Model file for the job. Use its own axes, mm. A direction names the side the tool comes from. Give positions to 0.01 mm unless a question says otherwise; leave off trailing zeros. Loops run counter-clockwise (first coordinate to the right, second up) from the corner with the lowest first, then second, coordinate; pieces in that order, holes last. Notation, with made-up numbers: M 89,32 L 105,32 A23 ccw 105,54 Z; hole C 0.5,64 d5. An arc over 180 degrees is marked long. Answer in a Markdown table with one row per item.
```python
from build123d import *

# Parameters (mm, degrees)
F0_R     = 2.55
F1_DEPTH = 5


with BuildPart() as f1:
    # F0 (on Top) → F1 (new body)
    with BuildSketch(Plane.XY):
        Polygon((-61.291651, 58.480762), (-81.291651, 23.839746), (-20, -11.547005), (-20, -82.320508), (20, -82.320508), (20, -11.547005), (81.291651, 23.839746), (61.291651, 58.480762), (0, 23.094011), align=None)
        with Locations((-10, -72.320508)):
            Circle(F0_R, mode=Mode.SUBTRACT)
        with Locations((-10, -32.320508)):
            Circle(F0_R, mode=Mode.SUBTRACT)
        with Locations((10, -72.320508)):
            Circle(F0_R, mode=Mode.SUBTRACT)
        with Locations((10, -32.320508)):
            Circle(F0_R, mode=Mode.SUBTRACT)
        with Locations((-67.631397, 27.5)):
            Circle(F0_R, mode=Mode.SUBTRACT)
        with Locations((-32.990381, 7.5)):
            Circle(F0_R, mode=Mode.SUBTRACT)
        with Locations((-22.990381, 24.820508)):
            Circle(F0_R, mode=Mode.SUBTRACT)
        with Locations((-57.631397, 44.820508)):
            Circle(F0_R, mode=Mode.SUBTRACT)
        with Locations((32.990381, 7.5)):
            Circle(F0_R, mode=Mode.SUBTRACT)
        with Locations((22.990381, 24.820508)):
            Circle(F0_R, mode=Mode.SUBTRACT)
        with Locations((67.631397, 27.5)):
            Circle(F0_R, mode=Mode.SUBTRACT)
        with Locations((57.631397, 44.820508)):
            Circle(F0_R, mode=Mode.SUBTRACT)
    extrude(amount=F1_DEPTH)


solid = f1.part
```
(1) Saw through at B-B, the plane x = 10. Give the cut face in (y, z), and give its area (3 significant figures).
Established:
| item | result |
|---|---|
| outline | M -82.32,0 L -74.87,0 L -74.87,5 L -82.32,5 Z; M -69.77,0 L -34.87,0 L -34.87,5 L -69.77,5 Z; M -29.77,0 L 28.87,0 L 28.87,5 L -29.77,5 Z |
| area | 505 mm2 |
(2) Saw through at D-D, the plane y = -54.5. Give the cut face in (x, z).
Established:
| item | result |
|---|---|
| outline | M -20,0 L 20,0 L 20,5 L -20,5 Z |
(3) Flat gauge pins, fed straight in: P1, Ø3, axis at y = 14, z = 3, coming from the +X side; P2, Ø1, axis at y = -8.5, z = 2, coming from the -X side; P3, Ø1, axis at x = -63.5, z = 3, coming from the +Y side. Where does each tip first touch, or does it go through?
Established:
| item | result |
|---|---|
| P1 | stops at x = 66.85 |
| P2 | stops at x = -26.14 |
| P3 | stops at y = 55.52 |
(4) Mould opens along Y. For faces 1 (the flat face through (20, -47, 2)), 2 (the cylindrical face through (-24.87, 26.544, 2.465)), 3 (the cylindrical face through (11.37, -70.17, 2.46)), 4 (the flat face through (50.22, 5.9, 2.46)) say: pulls with the +Y half, pulls with the -Y half, needs draft (parallel to the pull), parting line crosses it, or undercut.
Established:
| item | result |
|---|---|
| face 1 | needs draft |
| face 2 | undercut |
| face 3 | undercut |
| face 4 | pulls with the -Y half |
(5) Which spindle directions (+Z, -Z, +X, -X, +Y, -Y) get a long thin tool onto all of the face, cutting with end or side? Do faces 5 (the flat face through (-20, -46, 2)), 6 (the flat face through (71.43, 40.92, 2.46)), 7 (the flat face through (-30.22, 40.54, 2.46)). Say none if no direction does.
Established:
| item | result |
|---|---|
| face 5 | +Z, -Z, -X, -Y |
| face 6 | +Z, -Z, +X, +Y |
| face 7 | +Z, -Z, +Y |
(6) Saw through at C-C, the plane z = 2.3. Count the separate pieces of the cut face and the enclosed holes in it, and give its area (3 significant figures).
Established:
| item | result |
|---|---|
| separate pieces | 1 |
| enclosed holes | 12 |
| area | 8,940 mm2 |
(7) Wall check: L1, parallel to X at y = 23, z = 1.55; L2, parallel to Y at x = -12, z = 4.55; L3, parallel to X at y = -47, z = 2.1. Give the ranges that are in metal, low to high.
Established:
| item | result |
|---|---|
| L1 | x = -79.84 to -24.78, -21.2 to 21.2, 24.78 to 79.84 |
| L2 | y = -82.32 to -73.9, -70.74 to -33.9, -30.74 to 30.02 |
| L3 | x = -20 to 20 |
(8) Saw through at A-A, the plane y = 7.5. Give the cut face in (x, z).
Established:
| item | result |
|---|---|
| outline | M -52.99,0 L -35.54,0 L -35.54,5 L -52.99,5 Z; M -30.44,0 L 30.44,0 L 30.44,5 L -30.44,5 Z; M 35.54,0 L 52.99,0 L 52.99,5 L 35.54,5 Z |
